Design review of the part shown in the three views and the two pictorial views. Dimensions are in mm from the part's minimum x, y and z. Round coordinates to 2 decimals unless told otherwise and drop trailing zeros. Write each loop counter-clockwise with the first axis right and the second up, starting at its lowest first coordinate (ties: lowest second). Pieces come first, ordered by that corner, then holes. Notation, with made-up numbers: (64.25, -12) -> (110.25, -12) arc R33 ccw to (110.25, 25) -> close; hole circle Ø6 at (-14.5, -7). An arc over 180 degrees is marked (long way). Answer as a JSON object with one key per item and string values. Group by question number.
1) We need section A-A, the plane x = 27.5. Write out the cut boundary in (y, z), then the cut area to 4 significant figures.
2) We need section C-C, the plane x = 44. Write out the cut boundary in (y, z).
3) Insertion check: pin 1 Ø5.5 at (x, y) = (47.5, 37.5) entering from +Z; pin 2 Ø0.6 at (x, z) = (29.5, 4) entering from -Y; pin 3 Ø3 at (x, y) = (27.5, 37.5) entering from -Z. Each pin has a flat end and moves straight along its axis. Give the tip position at first contact, or say it passes through.
4) We need section B-B, the plane y = 37.5. Write out the cut boundary in (x, z), then the cut area to 3 significant figures.
5) To check wall thickness, follow probe 1 along X at (y, z) = (39, 4.6); probe 2 along Y at (x, z) = (27.5, 0.7). State the ranges of each line that lie inside material, in increasing order. Write a range as [from, to].
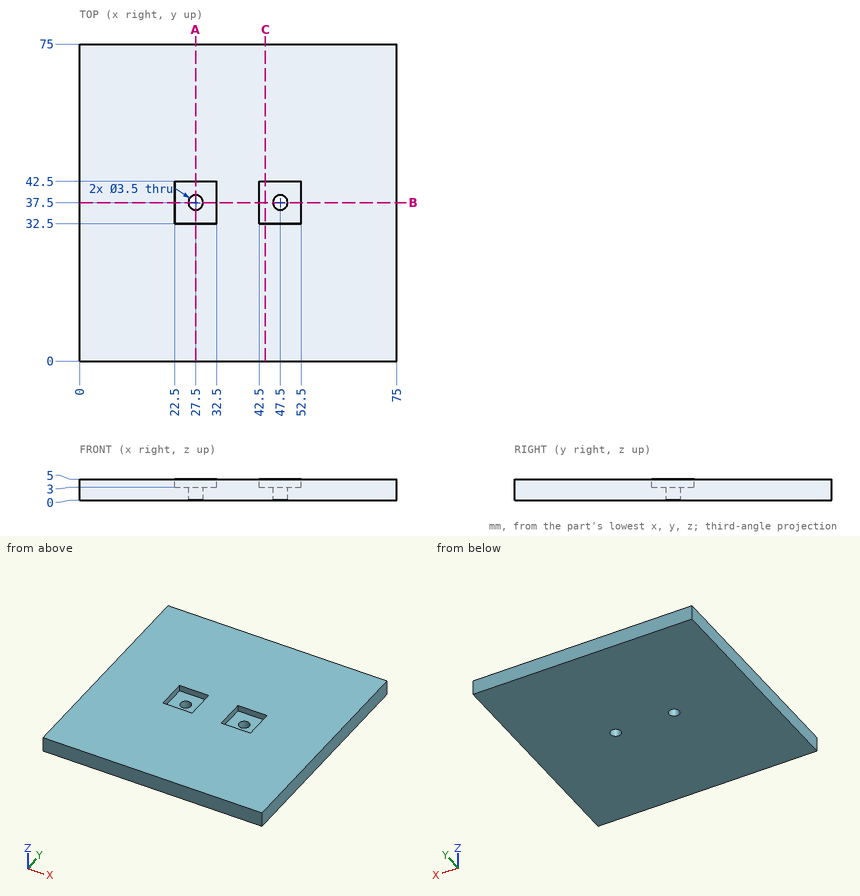
Here are the results:
{
 "1": {"outline": "(0, 0) -> (35.75, 0) -> (35.75, 3) -> (32.5, 3) -> (32.5, 5) -> (0, 5) -> close; (39.25, 0) -> (75, 0) -> (75, 5) -> (42.5, 5) -> (42.5, 3) -> (39.25, 3) -> close", "area": "344.5 mm^2"},
 "2": {"outline": "(0, 0) -> (75, 0) -> (75, 5) -> (42.5, 5) -> (42.5, 3) -> (32.5, 3) -> (32.5, 5) -> (0, 5) -> close"},
 "3": {"pin 1": "stops at z = 3", "pin 2": "stops at y = 0", "pin 3": "passes through"},
 "4": {"outline": "(0, 0) -> (25.75, 0) -> (25.75, 3) -> (22.5, 3) -> (22.5, 5) -> (0, 5) -> close; (29.25, 0) -> (45.75, 0) -> (45.75, 3) -> (42.5, 3) -> (42.5, 5) -> (32.5, 5) -> (32.5, 3) -> (29.25, 3) -> close; (49.25, 0) -> (75, 0) -> (75, 5) -> (52.5, 5) -> (52.5, 3) -> (49.25, 3) -> close", "area": "314 mm^2"},
 "5": {"probe 1": "x = [0, 22.5], [32.5, 42.5], [52.5, 75]", "probe 2": "y = [0, 35.75], [39.25, 75]"}
}
